Check sheet for the modelled part. Datum: model origin and axes. Units: mm. Round coordinates to 2 decimals unless told otherwise and drop trailing zeros. Write each loop counter-clockwise with the first axis right and the second up, starting at its lowest first coordinate (ties: lowest second). Pieces come first, ordered by that corner, then holes. Notation, with made-up numbers: M 21,17 L 47,17 A16 cw 47,36 Z; hole C 25,40.25 d1. An arc over 180 degrees is marked long. Put each result on its own line as item: value.
```python
from build123d import *

# Parameters (mm, degrees)
BOSS_EXTRUDE1_DEPTH      = 3
M4_CLEARANCE_HOLE1_D     = 4.5
M4_CLEARANCE_HOLE1_DEPTH = 12
M4_CLEARANCE_HOLE1_TIP   = 1.351936393


with BuildPart() as part:
    # Sketch1 → Boss-Extrude1 (new body)
    with BuildSketch(Plane(origin=(0, 0, 0), x_dir=(1, 0, 0), z_dir=(0, 1, 0))):
        Polygon((-112.62, 129), (-112.62, 0), (112.62, 0), (112.62, 129), (67.88, 129), (67.88, 108.5), (-88.12, 108.5), (-88.12, 129), align=None)
    extrude(amount=BOSS_EXTRUDE1_DEPTH)

    # M4 Clearance Hole1
    with Locations(Plane(origin=(0, 3, 0), x_dir=(1, 0, 0), z_dir=(0, 1, 0))):
        with Locations((-106.62, 5), (-106.62, 124), (109.12, 124), (109.12, 5)):
            Hole(M4_CLEARANCE_HOLE1_D / 2, depth=M4_CLEARANCE_HOLE1_DEPTH)
            with Locations((0, 0, -(M4_CLEARANCE_HOLE1_DEPTH + M4_CLEARANCE_HOLE1_TIP / 2))):  # 118° drill point
                Cone(0, M4_CLEARANCE_HOLE1_D / 2, M4_CLEARANCE_HOLE1_TIP, mode=Mode.SUBTRACT)


solid = part.part
```
1. Scan lines: probe 1 along Z at (x, y) = (109.12, 1.2); probe 2 along X at (y, z) = (1.3, -124); probe 3 along X at (y, z) = (2.6, -110.5). Record each from-to range of solid material in increasing order.
Computed values:
probe 1: z = -129 to -126.25, -121.75 to -7.25, -2.75 to 0
probe 2: x = -112.62 to -108.87, -104.37 to -88.12, 67.88 to 106.87, 111.37 to 112.62
probe 3: x = -112.62 to -88.12, 67.88 to 112.62
2. Cross-section at A-A (x = 109.12). Enter the section's corners in (y, z).
Computed values:
outline: M 0,-129 L 3,-129 L 3,-126.25 L 0,-126.25 Z; M 0,-121.75 L 3,-121.75 L 3,-7.25 L 0,-7.25 Z; M 0,-2.75 L 3,-2.75 L 3,0 L 0,0 Z
3. Cross-section at B-B (z = -5). Enter the section's corners in (x, y).
Computed values:
outline: M -112.62,0 L -108.87,0 L -108.87,3 L -112.62,3 Z; M -104.37,0 L 106.87,0 L 106.87,3 L -104.37,3 Z; M 111.37,0 L 112.62,0 L 112.62,3 L 111.37,3 Z
4. Depth check by flat-ended pin: pin 1 Ø1 at (x, y) = (-24.5, 1.5) entering from -Z; pin 2 Ø7 at (x, z) = (-106.62, -5) entering from -Y; pin 3 Ø2.5 at (x, z) = (109.12, -5) entering from -Y. Enter the tip coordinate at first touch or a pass-through.
Computed values:
pin 1: stops at z = -108.5
pin 2: stops at y = 0
pin 3: passes through
5. Cross-section at D-D (y = 2.4). Enter the section's corners in (x, z).
Computed values:
outline: M -112.62,-129 L -88.12,-129 L -88.12,-108.5 L 67.88,-108.5 L 67.88,-129 L 112.62,-129 L 112.62,0 L -112.62,0 Z; hole C -106.62,-124 d4.5; hole C -106.62,-5 d4.5; hole C 109.12,-124 d4.5; hole C 109.12,-5 d4.5
6. Release check for a two-part mould opening along Z. For faces 1 (the cylindrical face through (-108.7, 1.48, -123.14)), 2 (the flat face through (-2, 3, -65)), 3 (the cylindrical face through (-108.7, 1.48, -4.14)) record: +Z half, -Z half, draft (parallel to the pull), parting line (faces both ways), or undercut.
Computed values:
face 1: undercut
face 2: draft
face 3: undercut
7. Cross-section at C-C (z = -124). Enter the section's corners in (x, y).
Computed values:
outline: M -112.62,0 L -108.87,0 L -108.87,3 L -112.62,3 Z; M -104.37,0 L -88.12,0 L -88.12,3 L -104.37,3 Z; M 67.88,0 L 106.87,0 L 106.87,3 L 67.88,3 Z; M 111.37,0 L 112.62,0 L 112.62,3 L 111.37,3 Z
